Input: dimensioned drawing with shaded views. Units: mm. Origin: part minimum x, y, z. A direction names the side the tool comes from. Give positions to 0.01 mm unless a question says otherwise; leave off trailing zeros. Loops run counter-clockwise (first coordinate to the right, second up) from the corner with the lowest first, then second, coordinate; pieces in that order, holes last. Notation, with made-up numbers: M 24,51.5 L 43,51.5 A16 cw 43,58.5 Z; hole C 3.5,25 d6. An arc over 180 degrees is marked long. Answer in a Markdown table with one row per item.
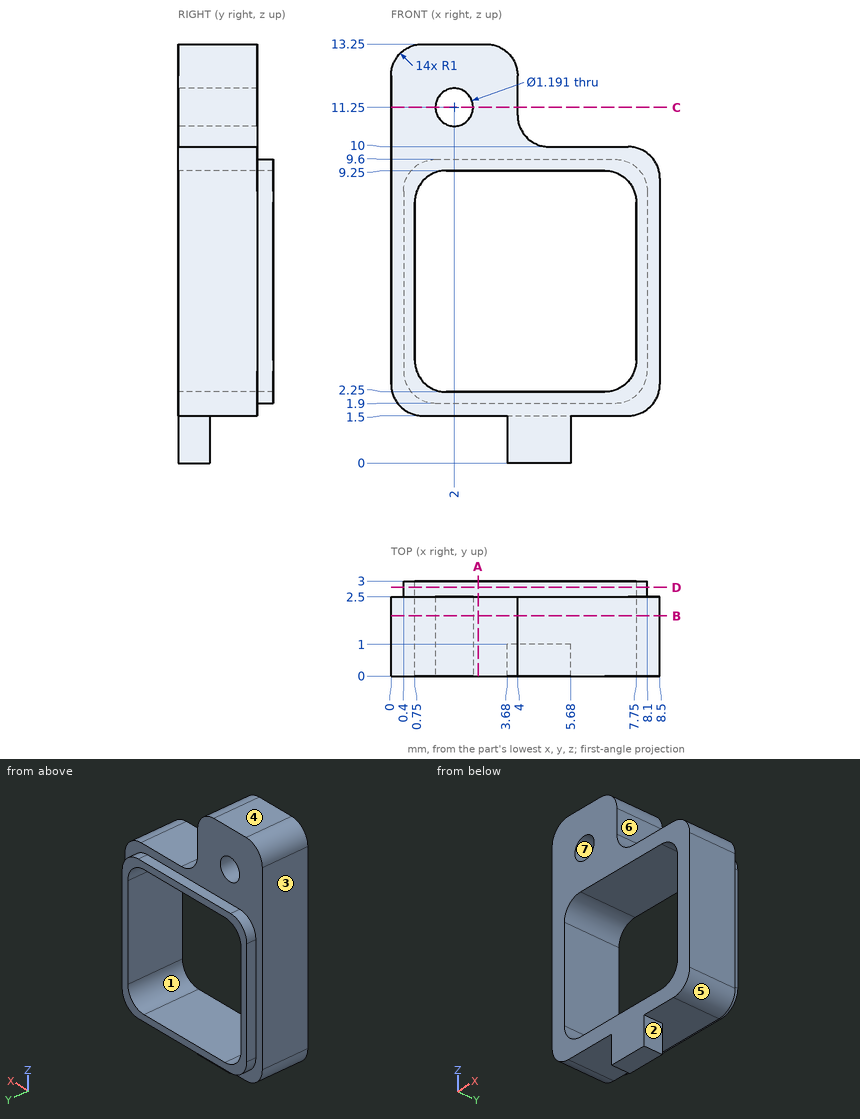
Q1. Reachability of the marked faces 1, 2 and 3 from +Z, -Z, +X, -X, +Y, -Y: full face, straight path, thin tool, end or side. Return the list, or none.
Values follow:
| item | result |
|---|---|
| face 1 | +Y, -Y |
| face 2 | -Z, +X, +Y, -Y |
| face 3 | +Z, -Z, -X, +Y, -Y |
Q2. Section query C-C (z = 11.25). Output: boundary loops of the cut face in (x, y) (1 decimal).
Values follow:
| item | result |
|---|---|
| outline | M 0,0 L 1.4,0 L 1.4,2.5 L 0,2.5 Z; M 2.6,0 L 4,0 L 4,2.5 L 2.6,2.5 Z |
Q3. Section query D-D (y = 2.8). Output: boundary loops of the cut face in (x, z).
Values follow:
| item | result |
|---|---|
| outline | M 0.4,2.9 A1 ccw 1.4,1.9 L 7.1,1.9 A1 ccw 8.1,2.9 L 8.1,8.6 A1 ccw 7.1,9.6 L 1.4,9.6 A1 ccw 0.4,8.6 Z; hole M 0.75,3.25 A1 ccw 1.75,2.25 L 6.75,2.25 A1 ccw 7.75,3.25 L 7.75,8.25 A1 ccw 6.75,9.25 L 1.75,9.25 A1 ccw 0.75,8.25 Z |
Q4. Section query A-A (x = 2.75). Output: boundary loops of the cut face in (y, z).
Values follow:
| item | result |
|---|---|
| outline | M 0,1.5 L 2.5,1.5 L 2.5,1.9 L 3,1.9 L 3,2.25 L 0,2.25 Z; M 0,9.25 L 3,9.25 L 3,9.6 L 2.5,9.6 L 2.5,13.25 L 0,13.25 Z |
Q5. Section query B-B (y = 1.9). Give the number of separate pieces and of enclosed holes in the cut face.
Values follow:
| item | result |
|---|---|
| separate pieces | 1 |
| enclosed holes | 2 |
Q6. Ray query, probe 1 along Z at (x, y) = (5.25, 1.05); probe 2 along X at (y, z) = (1.15, 11.25) (1 decimal); probe 3 along Z at (x, y) = (2, 2.65). Return the intervals inside material, ascending. Write a range as from..to.
Values follow:
| item | result |
|---|---|
| probe 1 | 1.5..2.25, 9.25..10 |
| probe 2 | 0..1.4, 2.6..4 |
| probe 3 | 1.9..2.25, 9.25..9.6 |
Q7. Contact query for flat-ended pins moving along their axis: pin 1 Ø4 at (x, z) = (2, 1.5) entering from -Y; pin 2 Ø0.8 at (x, z) = (4.5, 0.5) entering from +Y; pin 3 Ø1.5 at (x, z) = (2, 11.25) entering from +Y; pin 4 Ø1.4 at (y, z) = (0.5, 12) entering from +X. Output: stop coordinate, or through.
Values follow:
| item | result |
|---|---|
| pin 1 | y = 0 |
| pin 2 | y = 1 |
| pin 3 | y = 2.5 |
| pin 4 | x = 4 |
Q8. Mould query, pull axis Z, two halves, no side actions, for the marked faces 4, 5, 6 and 7. Classes: +Z half, -Z half, draft (parallel to the pull), parting line (faces both ways), or undercut.
Values follow:
| item | result |
|---|---|
| face 4 | +Z half |
| face 5 | -Z half |
| face 6 | draft |
| face 7 | undercut |
